The model under review builds one solid part; all positions refer to its coordinate system, in mm. Give positions to 0.01 mm unless a question says otherwise; leave off trailing zeros. Order: outer loops, then holes, each group sorted by start corner. A loop starts at its lowest first (then second) coordinate and runs counter-clockwise, first axis right, second up.
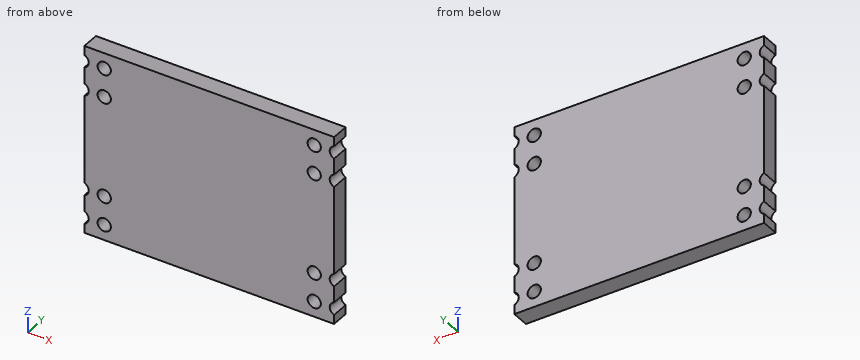
```python
from build123d import *

# Parameters (mm, degrees)
SKETCH1_W                       = 22.6
SKETCH1_H                       = 17.1
MAIN_BODY_DEPTH                 = 1.6
SKETCH2_R                       = 0.6
SOLDERED_CONNECTION_HOLES_DEPTH = 2.6
LPATTERN1_COUNT                 = 2
LPATTERN1_PITCH                 = 2
MIRROR1_COPY_1_SKETCH_R         = 0.6
MIRROR1_COPY_1_DEPTH            = 2.6
MIRROR2_COPY_1_SKETCH_R         = 0.6
MIRROR2_COPY_1_DEPTH            = 2.6
MIRROR2_COPY_2_SKETCH_R         = 0.6
MIRROR2_COPY_2_DEPTH            = 2.6
MIRROR2_COPY_3_SKETCH_R         = 0.6
MIRROR2_COPY_3_DEPTH            = 2.6


with BuildPart() as part:
    # Sketch1 → MAIN BODY (new body)
    with BuildSketch(Plane(origin=(0, 0, 0), x_dir=(1, 0, 0), z_dir=(0, 1, 0))):
        Rectangle(SKETCH1_W, SKETCH1_H)
    extrude(amount=MAIN_BODY_DEPTH)

    # Sketch2 → SOLDERED CONNECTION HOLES (cut, through all)
    with BuildSketch(Plane(origin=(0, 1.6, 0), x_dir=(1, 0, 0), z_dir=(0, 1, 0))):
        with Locations((-9.5, 7.15)):
            Circle(SKETCH2_R)
        with Locations((-9.5, 4.55)):
            Circle(SKETCH2_R)
    soldered_connection_holes = extrude(amount=-SOLDERED_CONNECTION_HOLES_DEPTH, mode=Mode.SUBTRACT)

    # LPattern1: SOLDERED CONNECTION HOLES ×2
    with Locations(*[(-i * LPATTERN1_PITCH, 0, 0) for i in range(1, LPATTERN1_COUNT)]):
        add(soldered_connection_holes, mode=Mode.SUBTRACT)

    # Mirror1: SOLDERED CONNECTION HOLES across plane
    add(soldered_connection_holes.mirror(Plane(origin=(0, 0, 0), x_dir=(0, 0, 1), z_dir=(1, 0, 0))), mode=Mode.SUBTRACT)

    # Mirror1 copy 1 sketch → Mirror1 copy 1 (cut, through all)
    with BuildSketch(Plane(origin=(2, 1.6, 0), x_dir=(-1, 0, 0), z_dir=(0, 1, 0))):
        with Locations((-9.5, -7.15)):
            Circle(MIRROR1_COPY_1_SKETCH_R)
        with Locations((-9.5, -4.55)):
            Circle(MIRROR1_COPY_1_SKETCH_R)
    extrude(amount=-MIRROR1_COPY_1_DEPTH, mode=Mode.SUBTRACT)

    # Mirror2: SOLDERED CONNECTION HOLES across plane
    add(soldered_connection_holes.mirror(Plane.XY), mode=Mode.SUBTRACT)

    # Mirror2 copy 1 sketch → Mirror2 copy 1 (cut, through all)
    with BuildSketch(Plane(origin=(-2, 1.6, 0), x_dir=(1, 0, 0), z_dir=(0, 1, 0))):
        with Locations((-9.5, -7.15)):
            Circle(MIRROR2_COPY_1_SKETCH_R)
        with Locations((-9.5, -4.55)):
            Circle(MIRROR2_COPY_1_SKETCH_R)
    extrude(amount=-MIRROR2_COPY_1_DEPTH, mode=Mode.SUBTRACT)

    # Mirror2 copy 2 sketch → Mirror2 copy 2 (cut, through all)
    with BuildSketch(Plane(origin=(0, 1.6, 0), x_dir=(-1, 0, 0), z_dir=(0, 1, 0))):
        with Locations((-9.5, 7.15)):
            Circle(MIRROR2_COPY_2_SKETCH_R)
        with Locations((-9.5, 4.55)):
            Circle(MIRROR2_COPY_2_SKETCH_R)
    extrude(amount=-MIRROR2_COPY_2_DEPTH, mode=Mode.SUBTRACT)

    # Mirror2 copy 3 sketch → Mirror2 copy 3 (cut, through all)
    with BuildSketch(Plane(origin=(2, 1.6, 0), x_dir=(-1, 0, 0), z_dir=(0, 1, 0))):
        with Locations((-9.5, 7.15)):
            Circle(MIRROR2_COPY_3_SKETCH_R)
        with Locations((-9.5, 4.55)):
            Circle(MIRROR2_COPY_3_SKETCH_R)
    extrude(amount=-MIRROR2_COPY_3_DEPTH, mode=Mode.SUBTRACT)


solid = part.part
```
Item 1: Clearance check with flat-ended pins moving along their axes: pin 1 Ø1.4 at (x, z) = (9.5, -4.55) entering from -Y; pin 2 Ø1 at (x, z) = (9.5, 7.15) entering from -Y. State where each tip first meets the part, or that it passes through.
Values found:
pin 1: stops at y = 0
pin 2: passes through
Item 2: Take a section at C-C (z = 7.15). Give the boundary of the cut face in (x, y).
Values found:
outline: (-10.9, 0) - (-10.1, 0) - (-10.1, 1.6) - (-10.9, 1.6) - close; (-8.9, 0) - (8.9, 0) - (8.9, 1.6) - (-8.9, 1.6) - close; (10.1, 0) - (10.9, 0) - (10.9, 1.6) - (10.1, 1.6) - close
Item 3: Take a section at B-B (y = 0.8). Give the number of separate pieces and of enclosed holes in the cut face, and give its area (3 significant figures).
Values found:
separate pieces: 1
enclosed holes: 8
area: 375 mm2
Item 4: For line 1 (X direction, y = 1.2, z = -4.55); line 2 (Z direction, x = -9.5, y = 0.7); line 3 (Z direction, x = -9, y = 1.35), list the stretches that pass through material, from the lowest coordinate up.
Values found:
line 1: x = -10.9 to -10.1, -8.9 to 8.9, 10.1 to 10.9
line 2: z = -8.55 to -7.75, -6.55 to -5.15, -3.95 to 3.95, 5.15 to 6.55, 7.75 to 8.55
line 3: z = -8.55 to -7.48, -6.82 to -4.88, -4.22 to 4.22, 4.88 to 6.82, 7.48 to 8.55
Item 5: Take a section at A-A (x = -9.5). Give the boundary of the cut face in (y, z), and give its area (3 significant figures).
Values found:
outline: (0, -8.55) - (1.6, -8.55) - (1.6, -7.75) - (0, -7.75) - close; (0, -6.55) - (1.6, -6.55) - (1.6, -5.15) - (0, -5.15) - close; (0, -3.95) - (1.6, -3.95) - (1.6, 3.95) - (0, 3.95) - close; (0, 5.15) - (1.6, 5.15) - (1.6, 6.55) - (0, 6.55) - close; (0, 7.75) - (1.6, 7.75) - (1.6, 8.55) - (0, 8.55) - close
area: 19.7 mm2
